Design review of the part built by this model. Coordinates are the model's own, in mm. A direction names the side the tool comes from. Coordinates: 2 decimals unless noted, no trailing zeros. Loops run counter-clockwise (first coordinate to the right, second up) from the corner with the lowest first, then second, coordinate; pieces in that order, holes last. Notation, with made-up numbers: (78.5, 74) - (90.5, 74) arc R7 ccw to (90.5, 81) - close; hole circle Ø4 at (36, 1). An arc over 180 degrees is marked (long way). Answer in a Markdown table with one row per item. Add a question column.
(1) For faces 1 (the face through (6, 0, -3)), 2 (the face through (-0.659, -1.715, 1.699)), 3 (the face through (7.969, 2.215, -2.699)), 4 (the face through (-10.04, 1.49, -5.34)), list the 3-axis set-ups (+Z, -Z, +X, -X, +Y, -Y) from which the entire face can be reached by the end or side of a thin tool; tool diameter is ignored.
(2) The part is to be moulded in two halves that separate along X. For faces 5 (the face through (10.25, 0, 0)), 6 (the face through (8, -2.5, 0)), 7 (the face through (5.75, 0, -2.7)), 8 (the face through (-1, 0, -2)), say which applies: released by +X, released by -X, zero draft, split by the parting line, or undercut.
(3) We need section B-B, the plane x = 2.25. Write out the cut boundary in (y, z), plus the area to 3 significant figures.
(4) We need section C-C, the plane z = 0. Write out the cut boundary in (x, y), plus the area to 3 significant figures.
(5) We need section A-A, the plane y = 0. Write out the cut boundary in (x, z), plus the area to 3 significant figures.
(6) Clearance check with flat-ended pins moving along their axes: pin 1 (1 mm diameter, centred on x = 3, y = -0.5, fed in from +Z); pin 2 (1 mm diameter, centred on x = -1.5, z = 0, fed in from -Y); pin 3 (1.5 mm diameter, centred on y = -1, z = -1.5, fed in from -X); pin 4 (1.8 mm diameter, centred on x = 8.25, y = 0, fed in from -Z). State where each tip first meets the part, or that it passes through.
(7) We need section D-D, the plane x = 7.5. Write out the cut boundary in (y, z).
(8) To check wall thickness, follow L1, parallel to Y at x = 8.25, z = 0.9; L2, parallel to X at y = 0, z = -1.85; L3, parallel to Y at x = -8.5, z = 2. State the ranges of each line that lie inside material, in increasing order. Write a range as [from, to].
from build123d import *

# Parameters (mm, degrees)
SKETCH_1_W                = 20.5
SKETCH_1_H                = 4
EXTRUDE_1_DEPTH           = 2
SKETCH_2_R                = 0.85
CUT_EXTRUDE_1_DEPTH       = 13
SKETCH_3_R                = 0.8
CUT_EXTRUDE_2_DEPTH       = 3
FILLET_1_R                = 1
SKETCH_4_W                = 4
SKETCH_4_H                = 4
CUT_EXTRUDE_5_DEPTH       = 1.5
CUT_EXTRUDE_6_DEPTH       = 1.5
SKETCH_7_W                = 1
SKETCH_7_H                = 4
EXTRUDE_2_DEPTH           = 1
FILLET_2_R                = 1
EXTRUDE_3_DEPTH           = 3
CUT_EXTRUDE_7_DEPTH       = 3
EXTRUDE_4_DEPTH           = 1
SKETCH_10_R               = 0.85
CUT_EXTRUDE_8_DEPTH       = 1
EXTRUDE_5_REACH           = 23.907
CUT_EXTRUDE_9_DEPTH       = 20.215826188
EXTRUDE_6_DEPTH           = 5
CUT_EXTRUDE_10_DEPTH      = 22.907341564
CUT_EXTRUDE_10_DEPTH_BACK = 22.907341564
SKETCH_14_R               = 1.5
FILLET_3_R                = 1


with BuildPart() as part:
    # 草图1 → 凸台-拉伸1 (new, symmetric)
    with BuildSketch(Plane.XY):
        Rectangle(SKETCH_1_W, SKETCH_1_H)
    extrude(amount=EXTRUDE_1_DEPTH, both=True)

    # 草图2 → 切除-拉伸1 (cut)
    with BuildSketch(Plane.XZ.offset(2)):
        with Locations(Location((-9.048459148, 0, 0), (0, 0, 270))):
            Circle(SKETCH_2_R)
    extrude(amount=-CUT_EXTRUDE_1_DEPTH, mode=Mode.SUBTRACT)

    # 草图3 → 切除-拉伸2 (cut)
    with BuildSketch(Plane.XY.offset(2)):
        with Locations((8.25, 0)):
            Circle(SKETCH_3_R)
    extrude(amount=-CUT_EXTRUDE_2_DEPTH, mode=Mode.SUBTRACT)

    # 圆角1
    fillet_1_edges = [part.edges().sort_by_distance(p)[0] for p in [
        (0, -2, 2),
        (0, -2, -2),
        (0, 2, -2),
        (0, 2, 2),
    ]]
    fillet(fillet_1_edges, radius=FILLET_1_R)

    # 草图4 → 切除-拉伸5 (cut)
    with BuildSketch(Plane.XZ.offset(2)):
        with Locations((-8.25, 0)):
            Rectangle(SKETCH_4_W, SKETCH_4_H)
    extrude(amount=-CUT_EXTRUDE_5_DEPTH, mode=Mode.SUBTRACT)

    # 草图5 → 切除-拉伸6 (cut)
    with BuildSketch(Plane(origin=(0, 2, 0), x_dir=(1, 0, 0), z_dir=(0, 1, 0))):
        Polygon((-6.25, 0), (-6.25, 2), (-10.25, 2), (-10.25, -2), (-6.25, -2), align=None)
    extrude(amount=-CUT_EXTRUDE_6_DEPTH, mode=Mode.SUBTRACT)

    # 草图7 → 凸台-拉伸2 (add)
    with BuildSketch(Plane.XZ.offset(0.5)):
        with Locations((-10.75, 0)):
            Rectangle(SKETCH_7_W, SKETCH_7_H)
    extrude(amount=-EXTRUDE_2_DEPTH)

    # 圆角2
    fillet_2_edges = [part.edges().sort_by_distance(p)[0] for p in [
        (-11.25, 0, 2),
        (-11.25, 0, -2),
    ]]
    fillet(fillet_2_edges, radius=FILLET_2_R)

    # 草图8 → 凸台-拉伸3 (add)
    with BuildSketch(Plane.XZ.offset(0.5)):
        with BuildLine():
            Line((-13.011033862, -8.830832343), (-6.991216755, -1.748643399))
            ThreePointArc((-6.991216755, -1.748643399), (-7.171159983, 1.940553489), (-10.864293035, 1.998186001))
            Line((-10.864293035, 1.998186001), (-17.742872996, -4.252662808))
            Line((-17.742872996, -4.252662808), (-18.461553282, -3.557322138))
            Line((-18.461553282, -3.557322138), (-11.537428317, 2.737705696))
            ThreePointArc((-11.537428317, 2.737705696), (-6.475862877, 2.659275921), (-6.229806023, -2.396913549))
            Line((-6.229806023, -2.396913549), (-12.292353576, -9.526173013))
            Line((-12.292353576, -9.526173013), (-13.011033862, -8.830832343))
        make_face()
    extrude(amount=-EXTRUDE_3_DEPTH)

    # 草图9 → 切除-拉伸7 (cut)
    with BuildSketch(Plane.XZ.offset(0.5)):
        with BuildLine():
            Line((-13.011033862, -8.830832343), (-6.989420262, -1.751365983))
            ThreePointArc((-6.989420262, -1.751365983), (-7.168982159, 1.942804723), (-10.867073667, 1.999891291))
            Line((-10.867073667, 1.999891291), (-17.742872996, -4.252662808))
            Line((-17.742872996, -4.252662808), (-13.011033862, -8.830832343))
        make_face()
    extrude(amount=-CUT_EXTRUDE_7_DEPTH, mode=Mode.SUBTRACT)

    # 草图9<2> → 凸台-拉伸4 (add)
    with BuildSketch(Plane.XZ.offset(0.5)):
        with BuildLine():
            Line((-13.011033862, -8.830832343), (-6.989420262, -1.751365983))
            ThreePointArc((-6.989420262, -1.751365983), (-7.168982159, 1.942804723), (-10.867073667, 1.999891291))
            Line((-10.867073667, 1.999891291), (-17.742872996, -4.252662808))
            Line((-17.742872996, -4.252662808), (-13.011033862, -8.830832343))
        make_face()
    extrude(amount=-EXTRUDE_4_DEPTH)

    # 草图10 → 切除-拉伸8 (cut)
    with BuildSketch(Plane(origin=(0, 0.5, 0), x_dir=(1, 0, 0), z_dir=(0, 1, 0))):
        with Locations(Location((-10.786836392, 1.796675975, 0), (0, 0, 270))):
            Circle(SKETCH_10_R)
        with Locations(Location((-12.525213635, 3.59335195, 0), (0, 0, 270))):
            Circle(SKETCH_10_R)
    extrude(amount=-CUT_EXTRUDE_8_DEPTH, mode=Mode.SUBTRACT)

    # 凸台-拉伸5: up to this face of the body (flat: up to its plane)
    extrude_5_end = Plane(part.part.faces().sort_by_distance((2.117336662, -0.003624728, -2))[0])
    # 草图11 → 凸台-拉伸5 (add, up to the picked face)
    with BuildSketch(Plane.XY.offset(2), mode=Mode.PRIVATE) as extrude_5_sk1:
        Polygon((-6.25, -2), (-6.25, -0.5), (-7.75, -0.5), align=None)
    extrude_5_tool1 = split(extrude(extrude_5_sk1.sketch, amount=-EXTRUDE_5_REACH, mode=Mode.PRIVATE), bisect_by=extrude_5_end, keep=Keep.BOTH, mode=Mode.PRIVATE)
    add(extrude_5_tool1.solids().sort_by(Axis((-6.75, -1, 2), (0, 0, -1)))[0])

    # 草图12 → 切除-拉伸9 (cut, through all)
    with BuildSketch(Plane(origin=(-6.25, 0, 0), x_dir=(0, 0, -1), z_dir=(1, 0, 0))):
        with BuildLine():
            Line((2, -1), (2, -2))
            Line((2, -2), (1, -2))
            ThreePointArc((1, -2), (1.707106781, -1.707106781), (2, -1))
        make_face()
        with BuildLine():
            Line((-1, -2), (-2, -2))
            Line((-2, -2), (-2, -1))
            ThreePointArc((-2, -1), (-1.707106781, -1.707106781), (-1, -2))
        make_face()
    extrude(amount=-CUT_EXTRUDE_9_DEPTH, mode=Mode.SUBTRACT)

    # 草图13 → 凸台-拉伸6 (add)
    with BuildSketch(Plane.XY.offset(2)):
        Polygon((10.25, -2), (10.25, 2.5), (5.75, 2.5), (5.75, -2.5), (10.25, -2.5), align=None)
    extrude(amount=-EXTRUDE_6_DEPTH)

    # 草图14 → 切除-拉伸10 (cut, two sides: drawn at the far end of the back side and taken through both)
    with BuildSketch(Plane.XY.offset(2).offset(-CUT_EXTRUDE_10_DEPTH_BACK)):
        with Locations((8.25, 0)):
            Circle(SKETCH_14_R)
    extrude(amount=CUT_EXTRUDE_10_DEPTH + CUT_EXTRUDE_10_DEPTH_BACK, mode=Mode.SUBTRACT)

    # 圆角3
    fillet_3_edges = [part.edges().sort_by_distance(p)[0] for p in [
        (8, 2.5, 2),
        (8, -2.5, 2),
        (8, 2.5, -3),
        (8, -2.5, -3),
    ]]
    fillet(fillet_3_edges, radius=FILLET_3_R)


solid = part.part
Responses:
| question | item | result |
|---|---|---|
| 1 | face 1 | -Z, +X, +Y, -Y |
| 1 | face 2 | +Z, -X, -Y |
| 1 | face 3 | -Z, +X, +Y |
| 1 | face 4 | +Y |
| 2 | face 5 | released by +X |
| 2 | face 6 | zero draft |
| 2 | face 7 | undercut |
| 2 | face 8 | undercut |
| 3 | outline | (-2, -1) arc R1 ccw to (-1, -2) - (1, -2) arc R1 ccw to (2, -1) - (2, 1) arc R1 ccw to (1, 2) - (-1, 2) arc R1 ccw to (-2, 1) - close |
| 3 | area | 15.1 mm2 |
| 4 | outline | (-14.55, -0.5) - (-7.75, -0.5) - (-6.25, -2) - (5.75, -2) - (5.75, -2.5) - (10.25, -2.5) - (10.25, 2.5) - (5.75, 2.5) - (5.75, 2) - (-5.35, 2) - (-5.35, 2.5) - (-6.35, 2.5) - (-6.35, 0.5) - (-13.07, 0.5) - (-13.07, 2.5) - (-14.55, 2.5) - close; hole circle Ø3 at (8.25, 0) |
| 4 | area | 76.5 mm2 |
| 5 | outline | (-18.46, -3.56) - (-12.29, -9.53) - (-6.23, -2.4) arc R3.7 ccw to (-5.94, -2) - (5.75, -2) - (5.75, -3) - (6.75, -3) - (6.75, 2) - (-5.94, 2) arc R3.7 ccw to (-11.54, 2.74) - close; (9.75, -3) - (10.25, -3) - (10.25, 2) - (9.75, 2) - close; hole circle Ø1.7 at (-12.53, -3.59); hole circle Ø1.7 at (-10.79, -1.8) |
| 5 | area | 142 mm2 |
| 6 | pin 1 | stops at z = 2 |
| 6 | pin 2 | stops at y = -2 |
| 6 | pin 3 | stops at x = -16.81 |
| 6 | pin 4 | passes through |
| 7 | outline | (-2.5, -2) arc R1 ccw to (-1.5, -3) - (-1.3, -3) - (-1.3, 2) - (-1.5, 2) arc R1 ccw to (-2.5, 1) - close; (1.3, -3) - (1.5, -3) arc R1 ccw to (2.5, -2) - (2.5, 1) arc R1 ccw to (1.5, 2) - (1.3, 2) - close |
| 8 | L1 | y = [-2.5, -1.5], [1.5, 2.5] |
| 8 | L2 | x = [-16.58, -11.64], [-9.94, 6.75], [9.75, 10.25] |
| 8 | L3 | y = [-0.5, 0.5] |
